The model under review builds one solid part; all positions refer to its coordinate system, in mm. Round coordinates to 2 decimals unless told otherwise and drop trailing zeros. Write each loop counter-clockwise with the first axis right and the second up, starting at its lowest first coordinate (ties: lowest second). Pieces come first, ordered by that corner, then holes. Notation, with made-up numbers: (60, 19.25) -> (105, 19.25) arc R19 ccw to (105, 48.25) -> close; hole circle Ø3 at (73, -2.5). An arc over 180 degrees is marked (long way). Answer as a JSON object with one key per item and string values. Group by question number.
1) We need section A-A, the plane y = -25. Write out the cut boundary in (x, z), then the cut area to 3 significant figures.
2) We need section C-C, the plane y = 15. Write out the cut boundary in (x, z).
3) To check wall thickness, follow probe 1 along Y at (x, z) = (-18, 1.75); probe 2 along Y at (x, z) = (-5, -3.5); probe 3 along Y at (x, z) = (15, 2). State the ranges of each line that lie inside material, in increasing order. Write a range as [from, to].
4) We need section B-B, the plane x = 55. Write out the cut boundary in (y, z), then the cut area to 3 significant figures.
5) Insertion check: pin 1 Ø2.5 at (x, y) = (-5, 10) entering from +Z. The pin has a flat end and moves straight along its axis. Give the tip position at first contact, or say it passes through.
6) We need section D-D, the plane x = -18. Write out the cut boundary in (y, z).
from build123d import *

# Parameters (mm, degrees)
SKETCH1_W             = 130
SKETCH1_H             = 60
BOSS_EXTRUDE1_DEPTH   = 6
M5X0_8_TAPPED_HOLE1_D = 4.2
M3X0_5_TAPPED_HOLE1_D = 2.5


with BuildPart() as part:
    # Sketch1 → Boss-Extrude1 (new body, symmetric)
    with BuildSketch(Plane.XY):
        Rectangle(SKETCH1_W, SKETCH1_H)
    extrude(amount=BOSS_EXTRUDE1_DEPTH, both=True)

    # M5x0.8 Tapped Hole1 (through all)
    with Locations(Plane.XY.offset(6)):
        with Locations((-18, 15), (-18, -5), (-5, 10), (35, 10)):
            Hole(M5X0_8_TAPPED_HOLE1_D / 2)

    # M3x0.5 Tapped Hole1 (through all)
    with Locations(Plane.XY.offset(6)):
        with Locations((15, -25), (55, -25)):
            Hole(M3X0_5_TAPPED_HOLE1_D / 2)


solid = part.part
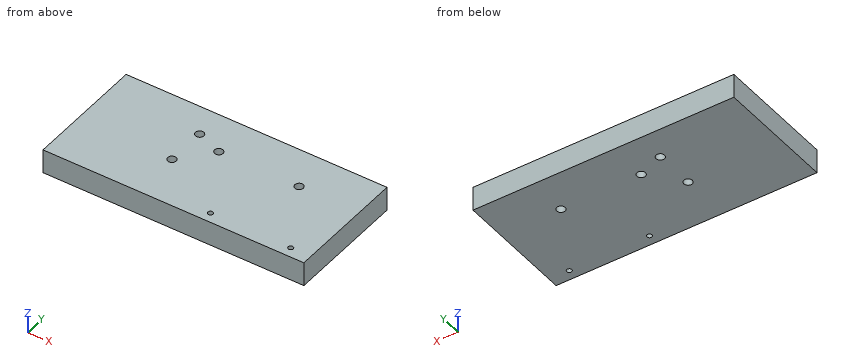
Here are the results:
{
 "1": {"outline": "(-65, -6) -> (13.75, -6) -> (13.75, 6) -> (-65, 6) -> close; (16.25, -6) -> (53.75, -6) -> (53.75, 6) -> (16.25, 6) -> close; (56.25, -6) -> (65, -6) -> (65, 6) -> (56.25, 6) -> close", "area": "1,500 mm^2"},
 "2": {"outline": "(-65, -6) -> (-20.1, -6) -> (-20.1, 6) -> (-65, 6) -> close; (-15.9, -6) -> (65, -6) -> (65, 6) -> (-15.9, 6) -> close"},
 "3": {"probe 1": "y = [-30, -7.1], [-2.9, 12.9], [17.1, 30]", "probe 2": "y = [-30, 7.9], [12.1, 30]", "probe 3": "y = [-30, -26.25], [-23.75, 30]"},
 "4": {"outline": "(-30, -6) -> (-26.25, -6) -> (-26.25, 6) -> (-30, 6) -> close; (-23.75, -6) -> (30, -6) -> (30, 6) -> (-23.75, 6) -> close", "area": "690 mm^2"},
 "5": {"pin 1": "passes through"},
 "6": {"outline": "(-30, -6) -> (-7.1, -6) -> (-7.1, 6) -> (-30, 6) -> close; (-2.9, -6) -> (12.9, -6) -> (12.9, 6) -> (-2.9, 6) -> close; (17.1, -6) -> (30, -6) -> (30, 6) -> (17.1, 6) -> close"}
}
